Geometry check sheet. Reference: drawing and pictorial views, mm from the part's lowest x, y, z. Give positions to 0.01 mm unless a question says otherwise; leave off trailing zeros. Order: outer loops, then holes, each group sorted by start corner. A loop starts at its lowest first (then second) coordinate and runs counter-clockwise, first axis right, second up. Notation, with made-up numbers: (44.5, 79) - (77.5, 79) arc R33 cw to (77.5, 109) - close; hole circle Ø4 at (69, -27.5). An arc over 180 degrees is marked (long way). Answer as a JSON object with one key per item and string values.
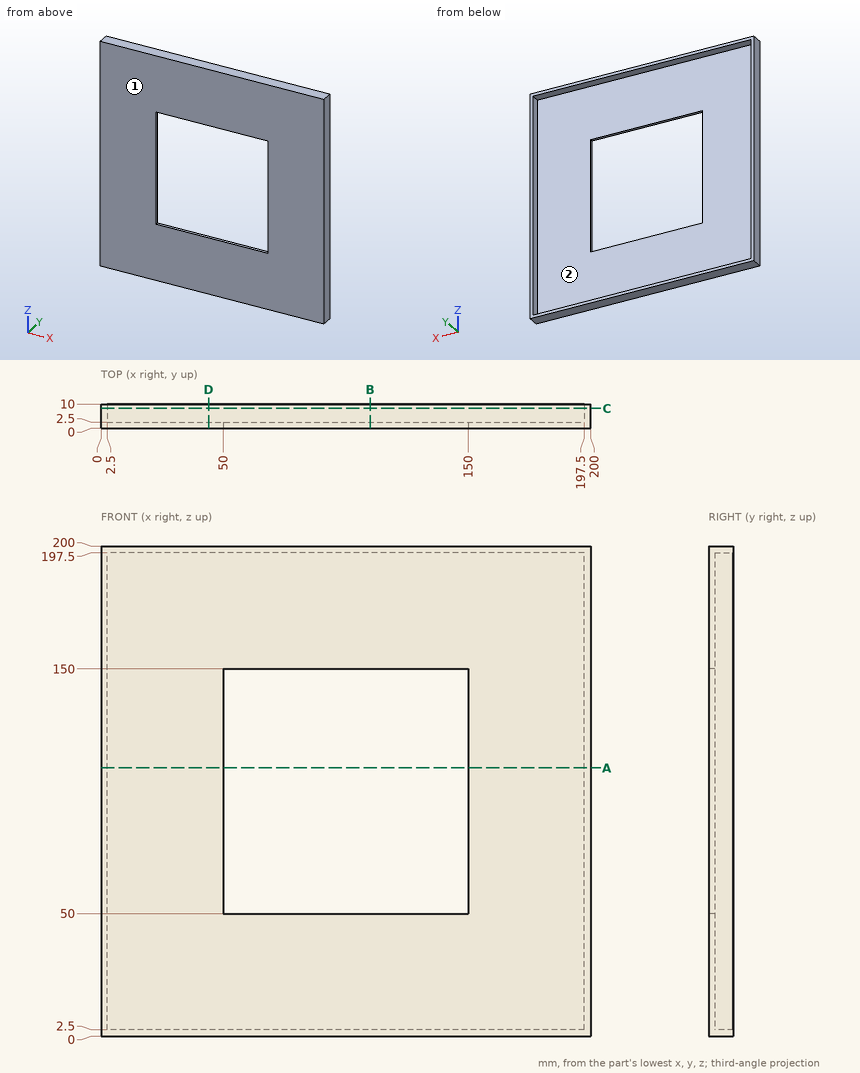
(1) Gauge pin test, flat end, axial feed: pin 1 Ø8 at (x, z) = (155.5, 67) entering from +Y. Record the tip position at first contact, or that the pin passes through.
Computed values:
{"pin 1": "stops at y = 2.5"}
(2) Section check C-C (y = 8.25). Record the cut outline in (x, z), then the cut area to 4 significant figures.
Computed values:
{"outline": "(0, 0) - (200, 0) - (200, 200) - (0, 200) - close; hole (2.5, 2.5) - (197.5, 2.5) - (197.5, 197.5) - (2.5, 197.5) - close", "area": "1,975 mm²"}
(3) Material ranges on line 1 along X through (y, z) = (2.75, 144); line 2 along X through (y, z) = (1.5, 90), recorded low to high. Write a range as [from, to].
Computed values:
{"line 1": "x = [0, 2.5], [197.5, 200]", "line 2": "x = [0, 50], [150, 200]"}
(4) Section check A-A (z = 109.5). Record the cut outline in (x, y).
Computed values:
{"outline": "(0, 0) - (50, 0) - (50, 2.5) - (2.5, 2.5) - (2.5, 10) - (0, 10) - close; (150, 0) - (200, 0) - (200, 10) - (197.5, 10) - (197.5, 2.5) - (150, 2.5) - close"}
(5) Section check B-B (x = 110). Record the cut outline in (y, z), then the cut area to 4 significant figures.
Computed values:
{"outline": "(0, 0) - (10, 0) - (10, 2.5) - (2.5, 2.5) - (2.5, 50) - (0, 50) - close; (0, 150) - (2.5, 150) - (2.5, 197.5) - (10, 197.5) - (10, 200) - (0, 200) - close", "area": "287.5 mm²"}
(6) Release check for a two-part mould opening along X. For the marked faces 1 and 2 record: pulls with the +X half, pulls with the -X half, needs draft (parallel to the pull), parting line crosses it, or undercut.
Computed values:
{"face 1": "needs draft", "face 2": "undercut"}
(7) Section check D-D (x = 44). Record the cut outline in (y, z), then the cut area to 4 significant figures.
Computed values:
{"outline": "(0, 0) - (10, 0) - (10, 2.5) - (2.5, 2.5) - (2.5, 197.5) - (10, 197.5) - (10, 200) - (0, 200) - close", "area": "537.5 mm²"}
